```python
from build123d import *

# Parameters (mm, degrees)
ESQUISSE1_R             = 5
SUPPORT_DEPTH           = 0.8
ESQUISSE2_R             = 5
BOUTON_DEPTH            = 6
CONG_1_R                = 0.5
ESQUISSE3_R             = 3.9
ENL_V_MAT_EXTRU_1_DEPTH = 5
DESSOUS_START           = 4.4
ESQUISSE4_R             = 0.85
DESSOUS_DEPTH           = 4.4


with BuildPart() as part:
    # Esquisse1 → Support (new body)
    with BuildSketch(Plane(origin=(0, 0, 0), x_dir=(1, 0, 0), z_dir=(0, 1, 0))):
        with BuildLine():
            Line((5.72974694, 0.9), (6.85, 0.9))
            ThreePointArc((6.85, 0.9), (7.063933825, 0.824394259), (7.182855864, 0.631154879))
            ThreePointArc((7.182855864, 0.631154879), (7.25, 0), (7.182855864, -0.631154879))
            ThreePointArc((7.182855864, -0.631154879), (7.063933825, -0.824394259), (6.85, -0.9))
            Line((6.85, -0.9), (5.72974694, -0.9))
            ThreePointArc((5.72974694, -0.9), (-5.8, 0), (5.72974694, 0.9))
        make_face()
        with Locations(Location((0, 0, 0), (0, 0, 270))):
            Circle(ESQUISSE1_R, mode=Mode.SUBTRACT)
    extrude(amount=SUPPORT_DEPTH)

    # Esquisse2 → Bouton (add)
    with BuildSketch(Plane(origin=(0, 0, 0), x_dir=(1, 0, 0), z_dir=(0, 1, 0))):
        with Locations(Location((0, 0, 0), (0, 0, 270))):
            Circle(ESQUISSE2_R)
    extrude(amount=BOUTON_DEPTH)

    # Congé1
    cong_1_edges = [part.edges().sort_by_distance(p)[0] for p in [
        (0, 6, -5),
    ]]
    fillet(cong_1_edges, radius=CONG_1_R)

    # Esquisse3 → Enlèv. mat.-Extru.1 (cut)
    with BuildSketch(Plane.XZ):
        with Locations(Location((0, 0, 0), (0, 0, 270))):
            Circle(ESQUISSE3_R)
    extrude(amount=-ENL_V_MAT_EXTRU_1_DEPTH, mode=Mode.SUBTRACT)

    # Esquisse4 → Dessous (add)
    with BuildSketch(Plane.XZ.offset(-5).offset(DESSOUS_START)):
        with BuildLine():
            Line((-0.5, 1.936491673), (-0.5, 3.867815921))
            ThreePointArc((-0.5, 3.867815921), (0, 3.9), (0.5, 3.867815921))
            Line((0.5, 3.867815921), (0.5, 1.936491673))
            ThreePointArc((0.5, 1.936491673), (1.414213562, 1.414213562), (1.936491673, 0.5))
            Line((1.936491673, 0.5), (3.867815921, 0.5))
            ThreePointArc((3.867815921, 0.5), (3.9, 0), (3.867815921, -0.5))
            Line((3.867815921, -0.5), (1.936491673, -0.5))
            ThreePointArc((1.936491673, -0.5), (1.414213562, -1.414213562), (0.5, -1.936491673))
            Line((0.5, -1.936491673), (0.5, -3.867815921))
            ThreePointArc((0.5, -3.867815921), (0, -3.9), (-0.5, -3.867815921))
            Line((-0.5, -3.867815921), (-0.5, -1.936491673))
            ThreePointArc((-0.5, -1.936491673), (-1.414213562, -1.414213562), (-1.936491673, -0.5))
            Line((-1.936491673, -0.5), (-3.867815921, -0.5))
            ThreePointArc((-3.867815921, -0.5), (-3.9, 0), (-3.867815921, 0.5))
            Line((-3.867815921, 0.5), (-1.936491673, 0.5))
            ThreePointArc((-1.936491673, 0.5), (-1.414213562, 1.414213562), (-0.5, 1.936491673))
        make_face()
        with Locations(Location((0, 0, 0), (0, 0, 270))):
            Circle(ESQUISSE4_R, mode=Mode.SUBTRACT)
    extrude(amount=-DESSOUS_DEPTH)


solid = part.part
```
CAD build for the part. Positions are in the model's coordinates, mm. A direction names the side the tool comes from. Coordinates: 2 decimals unless noted, no trailing zeros. Loops run counter-clockwise (first coordinate to the right, second up) from the corner with the lowest first, then second, coordinate; pieces in that order, holes last. Notation, with made-up numbers: (63, -27) - (87, -27) arc R25 ccw to (87, -9) - close; hole circle Ø10 at (-22, 20.5). An arc over 180 degrees is marked (long way). Use CSV: the item, a comma, the result in double quotes. Start each with the question number.
Q1. Two-plate mould, pull along X, no slides. Class faces 1 (the flat face through (4, 0, -1)), 2 (the cylindrical face through (-4.88, 3.12, -1.08)), 3 (the flat face through (-0.5, 3, -3)): +X half, -X half, draft (parallel to the pull), parting line (faces both ways), or undercut.
Q2. Cut at C-C, the plane y = 2.95. List the corners of the cut face in (x, z).
Q3. Probe probe 1 along Z at (x, y) = (3, 3.45); probe 2 along X at (y, z) = (4.05, 0). List the from-to ranges inside material, lowest first. Write a range as from..to.
Q4. Drop flat-ended pins along their axis: P1, Ø1, axis at x = 0, y = 3.5, coming from the +Z side; P2, Ø1, axis at x = -2.5, y = 3, coming from the -Z side; P3, Ø1.5, axis at y = 2.5, z = -3, coming from the -X side. Give the stop position or say it passes through.
Q5. Cut at D-D, the plane x = 6.25. List the corners of the cut face in (y, z).
Q6. Cut at B-B, the plane z = 0. List the corners of the cut face in (x, y).
Q7. Cut at A-A, the plane x = 0. List the corners of the cut face in (y, z), then the cut area to 3 significant figures.
Q8. 3-axis set-ups, long thin cutter, end or side, ignore diameter. For faces 4 (the flat face through (-0.5, 3, 3)), 5 (the cylindrical face through (-5.795, 0.394, 0.242)): which of +Z, -Z, +X, -X, +Y, -Y reach the whole face in a straight line?
Here are the results:
1,face 1,"draft"
1,face 2,"parting line"
1,face 3,"undercut"
2,outline,"circle Ø10 at (0, 0); hole (-3.87, -0.5) arc R3.9 ccw to (-0.5, -3.87) - (-0.5, -1.94) arc R2 cw to (-1.94, -0.5) - close; hole (-3.87, 0.5) - (-1.94, 0.5) arc R2 cw to (-0.5, 1.94) - (-0.5, 3.87) arc R3.9 ccw to start; hole circle Ø1.7 at (0, 0); hole (0.5, -3.87) arc R3.9 ccw to (3.87, -0.5) - (1.94, -0.5) arc R2 cw to (0.5, -1.94) - close; hole (0.5, 1.94) arc R2 cw to (1.94, 0.5) - (3.87, 0.5) arc R3.9 ccw to (0.5, 3.87) - close"
3,probe 1,"-4..-2.49, -0.5..0.5, 2.49..4"
3,probe 2,"-5..-0.85, 0.85..5"
4,P1,"z = 5"
4,P2,"z = -4.58"
4,P3,"x = -4.47"
5,outline,"(0, -0.9) - (0.8, -0.9) - (0.8, 0.9) - (0, 0.9) - close"
6,outline,"(-5.8, 0) - (-3.9, 0) - (-3.9, 0.6) - (-0.85, 0.6) - (-0.85, 5) - (0.85, 5) - (0.85, 0.6) - (3.9, 0.6) - (3.9, 0) - (7.25, 0) - (7.25, 0.8) - (5, 0.8) - (5, 5.5) arc R0.5 ccw to (4.5, 6) - (-4.5, 6) arc R0.5 ccw to (-5, 5.5) - (-5, 0.8) - (-5.8, 0.8) - close"
7,outline,"(0, -5.8) - (0.8, -5.8) - (0.8, -5) - (5.5, -5) arc R0.5 ccw to (6, -4.5) - (6, 4.5) arc R0.5 ccw to (5.5, 5) - (0.8, 5) - (0.8, 5.8) - (0, 5.8) - (0, 3.9) - (0.6, 3.9) - (0.6, 0.85) - (5, 0.85) - (5, -0.85) - (0.6, -0.85) - (0.6, -3.9) - (0, -3.9) - close"
7,area,"49.0 mm2"
8,face 4,"-Y"
8,face 5,"+Y, -Y"
